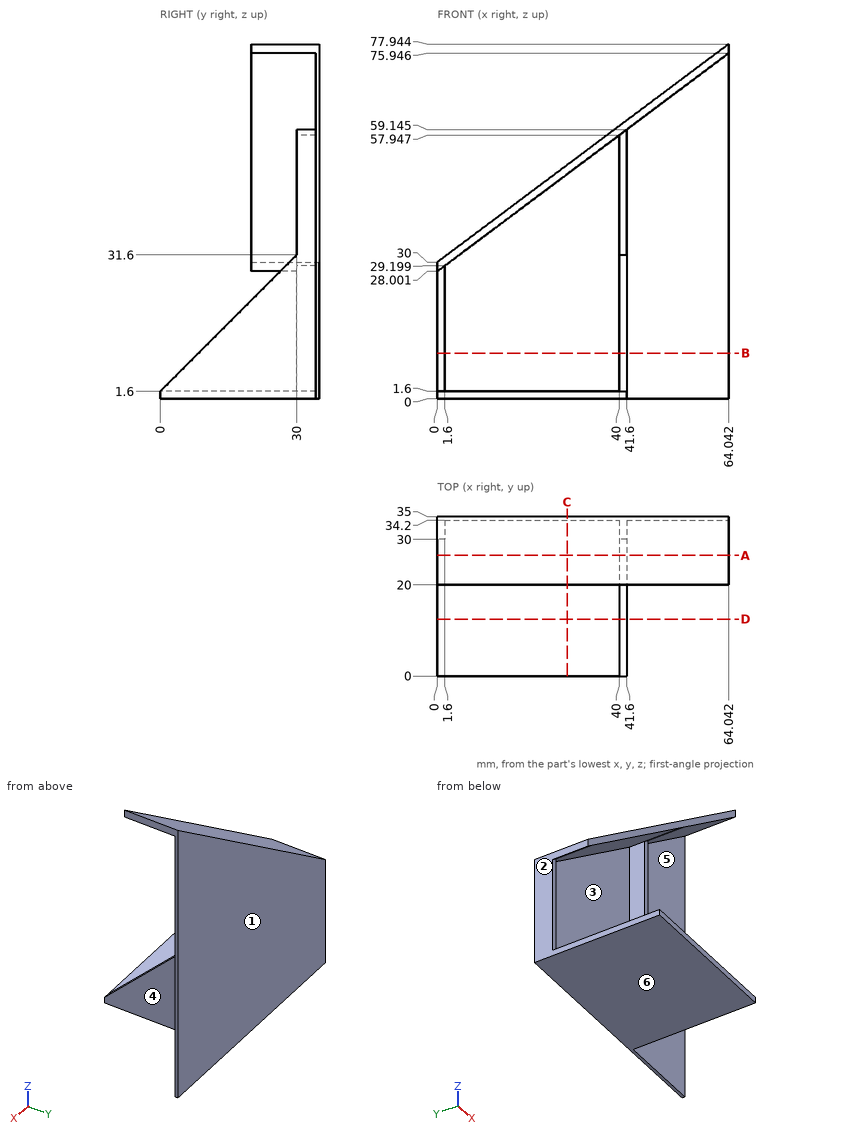
Design review of the part shown in the three views and the two pictorial views. Dimensions are in mm from the part's minimum x, y and z. A direction names the side the tool comes from. Coordinates: 2 decimals unless noted, no trailing zeros. Loops run counter-clockwise (first coordinate to the right, second up) from the corner with the lowest first, then second, coordinate; pieces in that order, holes last. Notation, with made-up numbers: (-21, 79.5) - (1, 79.5) arc R27 cw to (1, 104.5) - close; hole circle Ø4 at (11.5, -14). An arc over 180 degrees is marked (long way). Use a Markdown table: item, result. Add a question column.
Item 1: Insertion check: pin 1 Ø8 at (x, y) = (41, 23.5) entering from +Z; pin 2 Ø19 at (x, z) = (29.5, 21) entering from -Y; pin 3 Ø2 at (y, z) = (31, 20) entering from +X. Each pin has a flat end and moves straight along its axis. Give the tip position at first contact, or say it passes through.
Item 2: We need section C-C (x = 28.5). Give the boundary of the cut face in (y, z).
Item 3: Tool access review of the marked faces 5 and 6: name each direction out of +Z, -Z, +X, -X, +Y, -Y from which nothing blocks a thin tool from reaching the whole face with its end or side.
Item 4: We need section A-A (y = 26.5). Give the boundary of the cut face in (x, z) (1 decimal).
Item 5: We need section D-D (y = 12.5). Give the boundary of the cut face in (x, z).
Item 6: Mouldability with a two-part tool opening along X and no side actions: class the marked faces 1, 2, 3 and 4 as pulls with the +X half, pulls with the -X half, needs draft (parallel to the pull), parting line crosses it, or undercut.
Item 7: For line 1 (Z direction, x = 9, y = 11.5); line 2 (Y direction, x = 20, z = 6.5); line 3 (Z direction, x = 29, y = 23.5), list the stretches that pass through material, from the lowest coordinate up.
Item 8: We need section B-B (z = 10). Give the boundary of the cut face in (x, y).
Results list:
| question | item | result |
|---|---|---|
| 1 | pin 1 | stops at z = 63.69 |
| 1 | pin 2 | stops at y = 34.2 |
| 1 | pin 3 | stops at x = 41.6 |
| 2 | outline | (0, 0) - (35, 0) - (35, 51.34) - (20, 51.34) - (20, 49.34) - (34.2, 49.34) - (34.2, 1.6) - (0, 1.6) - close |
| 3 | face 5 | -Z, +X, -Y |
| 3 | face 6 | -Z, +X, -X, +Y, -Y |
| 4 | outline | (0, 0) - (41.6, 0) - (41.6, 28.1) - (40, 28.1) - (40, 1.6) - (0, 1.6) - close; (0, 28) - (40, 57.9) - (41.6, 59.1) - (64, 75.9) - (64, 77.9) - (0, 30) - close |
| 5 | outline | (0, 0) - (41.6, 0) - (41.6, 14.1) - (40, 14.1) - (40, 1.6) - (0, 1.6) - close |
| 6 | face 1 | needs draft |
| 6 | face 2 | pulls with the -X half |
| 6 | face 3 | undercut |
| 6 | face 4 | pulls with the +X half |
| 7 | line 1 | z = 0 to 1.6 |
| 7 | line 2 | y = 34.2 to 35 |
| 7 | line 3 | z = 0 to 1.6, 49.71 to 51.71 |
| 8 | outline | (0, 30) - (1.6, 30) - (1.6, 34.2) - (40, 34.2) - (40, 8.4) - (41.6, 8.4) - (41.6, 34.2) - (64.04, 34.2) - (64.04, 35) - (0, 35) - close |
